Input: part model. Units: mm. Frame: model coordinates. Round coordinates to 2 decimals unless told otherwise and drop trailing zeros. Order: outer loops, then holes, each group sorted by start corner. A loop starts at its lowest first (then second) coordinate and runs counter-clockwise, first axis right, second up. Notation, with made-up numbers: (-11, 54) -> (43, 54) arc R16 cw to (43, 81) -> close; hole circle Ø6 at (15.5, 26). An arc over 180 degrees is marked (long way). Use a Markdown table: item, result.
from build123d import *

# Parameters (mm, degrees)
SKETCH1_R           = 2.38125
SKETCH1_R_2         = 1.82245
BOSS_EXTRUDE1_DEPTH = 408.7876
SKETCH2_R           = 2.38125
BOSS_EXTRUDE2_DEPTH = 1.778
BOSS_EXTRUDE2_TAPER = -37
SKETCH3_R           = 1.82245
CUT_EXTRUDE1_DEPTH  = 2.7780001
CUT_EXTRUDE1_TAPER  = -37


with BuildPart() as part:
    # Sketch1 → Boss-Extrude1 (new body, symmetric)
    with BuildSketch(Plane.XY):
        Circle(SKETCH1_R)
        Circle(SKETCH1_R_2, mode=Mode.SUBTRACT)
    extrude(amount=BOSS_EXTRUDE1_DEPTH, both=True)

    # Sketch2 → Boss-Extrude2 (add)
    with BuildSketch(Plane.XY.offset(408.7876)):
        Circle(SKETCH2_R)
    boss_extrude2 = extrude(amount=BOSS_EXTRUDE2_DEPTH, taper=BOSS_EXTRUDE2_TAPER)

    # Sketch3 → Cut-Extrude1 (cut, through all)
    with BuildSketch(Plane(origin=(0, 0, 408.7876), x_dir=(-1, 0, 0), z_dir=(0, 0, -1))):
        Circle(SKETCH3_R)
    cut_extrude1 = extrude(amount=-CUT_EXTRUDE1_DEPTH, taper=CUT_EXTRUDE1_TAPER, mode=Mode.SUBTRACT)

    # Mirror1: Boss-Extrude2, Cut-Extrude1 across plane
    add(boss_extrude2.mirror(Plane.XY))
    add(cut_extrude1.mirror(Plane.XY), mode=Mode.SUBTRACT)


solid = part.part
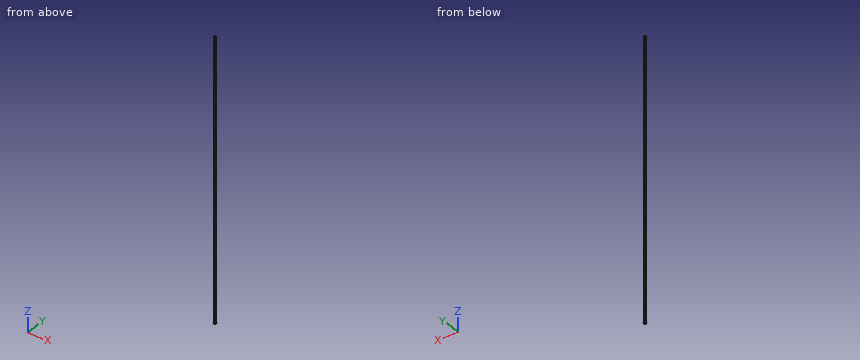
1) Ray query, probe 1 along Y at (x, z) = (0, 104.5); probe 2 along X at (y, z) = (-0.75, -188.5); probe 3 along X at (y, z) = (-0.5, 269). Return the intervals inside material, ascending.
Answer key:
| item | result |
|---|---|
| probe 1 | y = -2.38 to -1.82, 1.82 to 2.38 |
| probe 2 | x = -2.26 to -1.66, 1.66 to 2.26 |
| probe 3 | x = -2.33 to -1.75, 1.75 to 2.33 |
2) Cut plane B-B on z = 278. Return loops of the section in (x, y), and give its area (3 significant figures).
Answer key:
| item | result |
|---|---|
| outline | circle Ø4.76 at (0, 0); hole circle Ø3.64 at (0, 0) |
| area | 7.38 mm^2 |
3) Cut plane A-A on x = 0. Return loops of the section in (y, z).
Answer key:
| item | result |
|---|---|
| outline | (-3.72, -410.57) -> (-3.16, -410.57) -> (-1.82, -408.79) -> (-1.82, 408.79) -> (-3.16, 410.57) -> (-3.72, 410.57) -> (-2.38, 408.79) -> (-2.38, -408.79) -> close; (1.82, -408.79) -> (3.16, -410.57) -> (3.72, -410.57) -> (2.38, -408.79) -> (2.38, 408.79) -> (3.72, 410.57) -> (3.16, 410.57) -> (1.82, 408.79) -> close |
4) Contact query for flat-ended pins moving along their axis: P1, Ø1.5, axis at x = 1, z = 143.5, coming from the +Y side; P2, Ø2, axis at y = 3, z = 230.5, coming from the +X side; P3, Ø3, axis at x = 3, y = 0, coming from the +Z side; P4, Ø1.5, axis at x = -1.5, y = -1, coming from the +Z side. Output: stop coordinate, or through.
Answer key:
| item | result |
|---|---|
| P1 | stops at y = 2.37 |
| P2 | stops at x = 1.29 |
| P3 | stops at z = 410.57 |
| P4 | stops at z = 409.76 |
